Check sheet for the modelled part. Datum: model origin and axes. Units: mm. Give positions to 0.01 mm unless a question says otherwise; leave off trailing zeros. Order: outer loops, then holes, each group sorted by start corner. A loop starts at its lowest first (then second) coordinate and runs counter-clockwise, first axis right, second up.
Solid Edge part; units mm, degrees
sketch "Sketch1" plane through (0, 0, 0) normal (0, 0, 1) x (1, 0, 0)
  line L0 (120, 110) -> (0, 110)
  line L1 (0, 110) -> (0, 0)
  line L2 (0, 0) -> (120, 0)
  line L3 (120, 0) -> (120, 110)
extrude "Protrusion1" add sketch "Sketch1" along normal blind 5
sketch "Sketch2" plane through (60, 20, 5) normal (0, 0, 1) x (1, 0, 0)
  line L0 (55, -20) -> (55, 90)
  line L1 (55, 90) -> (60, 90)
  line L2 (60, 90) -> (60, -20)
  line L3 (60, -20) -> (55, -20)
  line L4 (-55, 90) -> (-55, -20)
  line L5 (-55, -20) -> (-60, -20)
  line L6 (-60, -20) -> (-60, 90)
  line L7 (-60, 90) -> (-55, 90)
extrude "Extrusionsausprägung_2" add sketch "Sketch2" along normal blind 80
hole "Bohrung_1" at (120, 20, 45) direction (-1, 0, 0) diameter 19 end up to next
hole "Hole_2" at (20, 10, 5) direction (0, 0, -1) diameter 4.2 end up to next start chamfer 0.6 start chamfer angle 45
hole "Hole1" at (20, 100, 5) direction (0, 0, -1) diameter 4.2 end up to next start chamfer 0.6 start chamfer angle 45
hole "Hole2" at (40, 100, 5) direction (0, 0, -1) diameter 4.2 end up to next start chamfer 0.6 start chamfer angle 45
hole "Hole3" at (40, 10, 5) direction (0, 0, -1) diameter 4.2 end up to next start chamfer 0.6 start chamfer angle 45
hole "Hole4" at (0, 20, 45) direction (1, 0, 0) diameter 8 end up to next
hole "Hole5" at (120, 65, 45) direction (-1, 0, 0) diameter 8 end up to next
sketch "Sketch3" plane through (60, 0, 42.5) normal (0, -1, 0) x (1, 0, 0)
  line L0 (55, -37.5) -> (55, 42.5)
  line L1 (55, 42.5) -> (60, 42.5)
  line L2 (60, 42.5) -> (60, -37.5)
  line L3 (60, -37.5) -> (55, -37.5)
  line L4 (-55, -37.5) -> (-60, -37.5)
  line L5 (-60, -37.5) -> (-60, 42.5)
  line L6 (-60, 42.5) -> (-55, 42.5)
  line L7 (-55, 42.5) -> (-55, -37.5)
extrude "Cutout1" cut sketch "Sketch3" against normal up to next
hole "Hole6" at (4, 10, 5) direction (0, 0, -1) diameter 4.1 end up to next
hole "Hole7" at (116, 10, 5) direction (0, 0, -1) diameter 4.1 end up to next
hole "Hole8" at (116, 100, 5) direction (0, 0, -1) diameter 4.1 end up to next
hole "Hole9" at (4, 100, 5) direction (0, 0, -1) diameter 4.1 end up to next
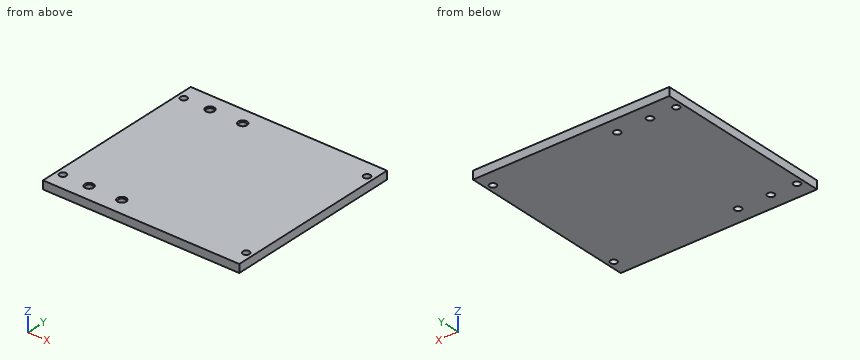
(1) Cross-section at B-B on x = 116. Enter the section's corners in (y, z).
Response values:
outline: (0, 0) - (7.95, 0) - (7.95, 5) - (0, 5) - close; (12.05, 0) - (97.95, 0) - (97.95, 5) - (12.05, 5) - close; (102.05, 0) - (110, 0) - (110, 5) - (102.05, 5) - close
(2) Cross-section at C-C on x = 40. Enter the section's corners in (y, z), then the cut area to 3 significant figures.
Response values:
outline: (0, 0) - (7.9, 0) - (7.9, 4.4) - (7.3, 5) - (0, 5) - close; (12.1, 0) - (97.9, 0) - (97.9, 4.4) - (97.3, 5) - (12.7, 5) - (12.1, 4.4) - close; (102.1, 0) - (110, 0) - (110, 5) - (102.7, 5) - (102.1, 4.4) - close
area: 507 mm2
(3) Cross-section at A-A on y = 100. Enter the section's corners in (x, z).
Response values:
outline: (0, 0) - (1.95, 0) - (1.95, 5) - (0, 5) - close; (6.05, 0) - (17.9, 0) - (17.9, 4.4) - (17.3, 5) - (6.05, 5) - close; (22.1, 0) - (37.9, 0) - (37.9, 4.4) - (37.3, 5) - (22.7, 5) - (22.1, 4.4) - close; (42.1, 0) - (113.95, 0) - (113.95, 5) - (42.7, 5) - (42.1, 4.4) - close; (118.05, 0) - (120, 0) - (120, 5) - (118.05, 5) - close
(4) Gauge pin test, flat ends, axial feed: pin 1 Ø3.5 at (x, y) = (20, 100) entering from +Z; pin 2 Ø5 at (x, y) = (40, 10) entering from +Z. Record the tip position at first contact, or that the pin passes through.
Response values:
pin 1: passes through
pin 2: stops at z = 4.8
(5) Material ranges on L1, parallel to X at y = 100, z = 1.65; L2, parallel to Y at x = 20, z = 2.05; L3, parallel to Y at x = 4, z = 3.55, recorded low to high.
Response values:
L1: x = 0 to 1.95, 6.05 to 17.9, 22.1 to 37.9, 42.1 to 113.95, 118.05 to 120
L2: y = 0 to 7.9, 12.1 to 97.9, 102.1 to 110
L3: y = 0 to 7.95, 12.05 to 97.95, 102.05 to 110
